from build123d import *

# Parameters (mm, degrees)
SKETCH1_W           = 150
SKETCH1_H           = 8
SKETCH1_R           = 2.75
BOSS_EXTRUDE1_DEPTH = 40
SKETCH2_R           = 1.5
CUT_EXTRUDE1_DEPTH  = 86.375640554
SKETCH3_W           = 40
SKETCH3_H           = 35
SKETCH3_H_2         = 25
CUT_EXTRUDE2_DEPTH  = 86.375640554
FILLET1_R           = 5
SKETCH4_R           = 2.5
CUT_EXTRUDE3_DEPTH  = 86.375640554
SKETCH5_R           = 1.5
BOSS_EXTRUDE2_DEPTH = 5


with BuildPart() as part:
    # Sketch1 → Boss-Extrude1 (new, symmetric)
    with BuildSketch(Plane(origin=(0, 0, 0), x_dir=(1, 0, 0), z_dir=(0, 1, 0))):
        Rectangle(SKETCH1_W, SKETCH1_H)
        with Locations(Location((-65.125, 0, 0), (0, 0, 270))):
            Circle(SKETCH1_R, mode=Mode.SUBTRACT)
        with Locations(Location((65.125, 0, 0), (0, 0, 270))):
            Circle(SKETCH1_R, mode=Mode.SUBTRACT)
    extrude(amount=BOSS_EXTRUDE1_DEPTH, both=True)

    # Sketch2 → Cut-Extrude1 (cut, through all)
    with BuildSketch(Plane.XY.offset(4)):
        with Locations((-18.75, 18.75)):
            Circle(SKETCH2_R)
        with Locations((18.75, 18.75)):
            Circle(SKETCH2_R)
        with Locations((18.75, -18.75)):
            Circle(SKETCH2_R)
        with Locations((-18.75, -18.75)):
            Circle(SKETCH2_R)
    extrude(amount=-CUT_EXTRUDE1_DEPTH, mode=Mode.SUBTRACT)

    # Sketch3 → Cut-Extrude2 (cut, through all)
    with BuildSketch(Plane.XY.offset(4)):
        with Locations((-55, 0)):
            Rectangle(SKETCH3_W, SKETCH3_H)
        with Locations((55, 27.5)):
            Rectangle(SKETCH3_W, SKETCH3_H_2)
        with Locations((55, -27.5)):
            Rectangle(SKETCH3_W, SKETCH3_H_2)
    extrude(amount=-CUT_EXTRUDE2_DEPTH, mode=Mode.SUBTRACT)

    # Fillet1
    fillet1_edges = [part.edges().sort_by_distance(p)[0] for p in [
        (-75, 40, 0),
        (-75, -17.5, 0),
        (-75, 17.5, 0),
        (-35, 17.5, 0),
        (-35, -17.5, 0),
        (-75, -40, 0),
        (75, 15, 0),
        (35, 15, 0),
        (35, 40, 0),
        (35, -15, 0),
        (75, -15, 0),
        (35, -40, 0),
    ]]
    fillet(fillet1_edges, radius=FILLET1_R)

    # Sketch4 → Cut-Extrude3 (cut, through all)
    with BuildSketch(Plane.XY.offset(4)):
        Circle(SKETCH4_R)
    extrude(amount=-CUT_EXTRUDE3_DEPTH, mode=Mode.SUBTRACT)

    # Sketch5 → Boss-Extrude2 (add)
    with BuildSketch(Plane.XY.offset(4)):
        with Locations(Location((10, 3, 0), (0, 0, 180))):
            Circle(SKETCH5_R)
    extrude(amount=BOSS_EXTRUDE2_DEPTH)


solid = part.part
Can you work these out from the model? Positions are in its coordinate system, mm. A direction names the side the tool comes from. Round coordinates to 2 decimals unless told otherwise and drop trailing zeros. Loops run counter-clockwise (first coordinate to the right, second up) from the corner with the lowest first, then second, coordinate; pieces in that order, holes last. Notation, with made-up numbers: (80.5, 26.25) - (116.5, 26.25) arc R23 ccw to (116.5, 37.25) - close; hole circle Ø1 at (-22.5, 26.5). An arc over 180 degrees is marked (long way). Answer in a Markdown table with one row per item. Add a question column.
Q1. I want a section at A-A on x = -18.75. List the corners of the cut face in (y, z) for me.
Q2. For pin 1 Ø1 at (x, y) = (15, 4.5) entering from +Z; pin 2 Ø3 at (x, y) = (0, 0) entering from +Z; pin 3 Ø2.5 at (x, z) = (58, 1.5) entering from +Y; pin 4 Ø7 at (x, z) = (65.125, 0) entering from -Y, each with a flat end and sliding along its axis, tell me the tip position at first contact or that it passes through.
Q3. I need wall thicknesses on L1, parallel to Y at x = -18.75, z = -0.25; L2, parallel to Y at x = -17.5, z = -1; L3, parallel to X at y = 24, z = 1.5. Which ranges of each line are inside material? Lowest first, please.
Q4. We'd pull the mould along Y, two halves only. Please class faces 5 (the cylindrical face through (33, 39, 0)), 6 (the cylindrical face through (37, -16, 0)), 7 (the cylindrical face through (-20.25, -18.68, 0.06)): pulls with the +Y half, pulls with the -Y half, needs draft (parallel to the pull), parting line crosses it, or undercut.
Q5. I want a section at C-C on x = -45. List the corners of the cut face in (y, z) for me, and give its area (3 significant figures).
Q6. I want a section at B-B on y = 0. List the corners of the cut face in (x, z) for me (3 decimals), and give its area (3 significant figures).
Q7. Which directions (+Z, -Z, +X, -X, +Y, -Y) give clear straight access to the entire face, cutting with the end or side of a thin tool? Please do faces 1 (the cylindrical face through (11.11, 1.99, 6.46)), 2 (the flat face through (35, -28, 0)), 3 (the cylindrical face through (-73.5, 18.93, -0.06)), 4 (the flat face through (55, 15, 0)).
Q8. I want a section at D-D on z = 0. Count the separate pieces of the cut face and the enclosed holes in it, and give its area (3 significant figures).
A:
| question | item | result |
|---|---|---|
| 1 | outline | (-40, -4) - (-20.25, -4) - (-20.25, 4) - (-40, 4) - close; (-17.25, -4) - (17.25, -4) - (17.25, 4) - (-17.25, 4) - close; (20.25, -4) - (40, -4) - (40, 4) - (20.25, 4) - close |
| 2 | pin 1 | z = 4 |
| 2 | pin 2 | through |
| 2 | pin 3 | y = 15 |
| 2 | pin 4 | y = -15 |
| 3 | L1 | -40 to -20.25, -17.25 to 17.25, 20.25 to 40 |
| 3 | L2 | -40 to -19.58, -17.92 to 17.92, 19.58 to 40 |
| 3 | L3 | -75 to -67.43, -62.82 to 35 |
| 4 | face 5 | pulls with the +Y half |
| 4 | face 6 | pulls with the -Y half |
| 4 | face 7 | undercut |
| 5 | outline | (-40, -4) - (-17.5, -4) - (-17.5, 4) - (-40, 4) - close; (17.5, -4) - (40, -4) - (40, 4) - (17.5, 4) - close |
| 5 | area | 360 mm^2 |
| 6 | outline | (-35, -4) - (-2.5, -4) - (-2.5, 4) - (-35, 4) - close; (2.5, -4) - (75, -4) - (75, 4) - (2.5, 4) - close; hole circle Ø5.5 at (65.125, 0) |
| 6 | area | 816 mm^2 |
| 7 | face 1 | +Z |
| 7 | face 2 | +Z, -Z, +X, -Y |
| 7 | face 3 | +Z, -Z, -X |
| 7 | face 4 | +Z, -Z, +X, +Y |
| 8 | separate pieces | 4 |
| 8 | enclosed holes | 5 |
| 8 | area | 8,120 mm^2 |
